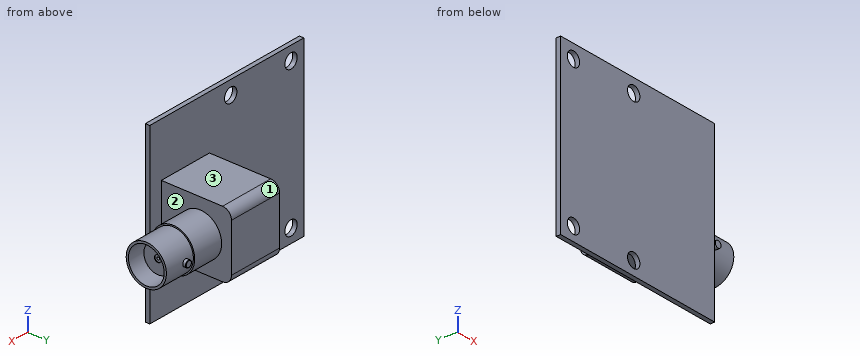
Autodesk Inventor part; units mm, degrees
ref_plane "YZ Plane" through (0, 0, 0) normal (1, 0, 0) x (0, 1, 0)
ref_plane "XZ Plane" through (0, 0, 0) normal (0, 1, 0) x (-1, 0, 0)
ref_plane "XY Plane" through (0, 0, 0) normal (0, 0, 1) x (1, 0, 0)
sketch "Sketch1" plane through (0, 0, 0) normal (0, 1, 0) x (-1, 0, 0)
  line L0 (0, 0) -> (40, 0)
  line L1 (40, 0) -> (40, -38.6)
  line L2 (40, -38.6) -> (0, -38.6)
  line L3 (0, -38.6) -> (0, 0)
  dimension "d0" = 40
  dimension "d1" = 38.6
extrude "Extrusion1" add sketch "Sketch1" along normal blind 1
sketch "Sketch6" plane through (0, 1, 0) normal (0, 1, 0) x (1, 0, 0)
  circle A0 centre (-36.676, 3.059) radius 1.6
  circle A1 centre (-21.026, 3.059) radius 1.6
  circle A2 centre (-21.026, 35.541) radius 1.6
  circle A3 centre (-36.676, 35.541) radius 1.6
  line L0 (0, 38.6) -> (-40, 38.6)
  line L1 (-40, 38.6) -> (-40, 0)
  point P0 (0, 0)
  dimension "d35" = 3.2
  dimension "d36" = 3.2
  dimension "d37" = 3.2
  dimension "d38" = 3.2
  dimension "d39" = 15.65
  dimension "d40" = 15.65
  dimension "d41" = 32.482
  dimension "d42" = 0
  dimension "d43" = 0
  dimension "d44" = 0
  dimension "d45" = 3.059
  dimension "d46" = 3.324
extrude "Extrusion5" cut sketch "Sketch6" against normal blind 5
sketch "Sketch7" plane through (0, 1, 0) normal (0, 1, 0) x (1, 0, 0)
  line L0 (-15.5, 26.65) -> (-3, 26.65)
  line L1 (-3, 26.65) -> (-3, 11.95)
  line L2 (-3, 11.95) -> (-15.5, 11.95)
  line L3 (-15.5, 11.95) -> (-15.5, 26.65)
  line L4 (0, 38.6) -> (-40, 38.6)
  line L5 (0, 0) -> (0, 38.6)
  dimension "d49" = 12.5
  dimension "d50" = 14.7
  dimension "d51" = 11.95
  dimension "d52" = 3
extrude "Extrusion6" add sketch "Sketch7" along normal blind 15.7
sketch "Sketch9" plane through (-3, 1, -11.95) normal (1, 0, 0) x (0, 0, -1)
  circle A0 centre (7.35, 8.7) radius 4.8
  line L0 (14.7, 0) -> (14.7, 15.7)
  line L1 (0, 15.7) -> (14.7, 15.7)
  point P0 (-11.95, -1)
  dimension "d55" = 9.6
  dimension "d56" = 7.35
  dimension "d57" = 7
extrude "Extrusion7" add sketch "Sketch9" along normal blind 7
fillet "Fillet1" radius 2 2 edges at (-9.25, 16.7, -11.95) (-9.25, 16.7, -26.65)
sketch "Sketch10" plane through (4, 9.7, -19.3) normal (1, 0, 0) x (0, 0, -1)
  circle A0 centre (0, 0) radius 4.5
  line L0 (7.35, -8.7) -> (7.35, 5)
  line L1 (-5.35, 7) -> (5.35, 7)
  point P0 (-19.3, -9.7)
  dimension "d61" = 9
  dimension "d62" = 7.35
  dimension "d63" = 7
extrude "Extrusion8" add sketch "Sketch10" along normal blind 7
sketch "Sketch11" plane through (11, 9.7, -19.3) normal (1, 0, 0) x (0, 0, -1)
  circle A0 centre (0, 0) radius 4
  point P0 (-19.3, -9.7)
  dimension "d66" = 8
extrude "Extrusion9" cut sketch "Sketch11" against normal blind 10
sketch "Sketch12" plane through (1, 9.7, -19.3) normal (1, 0, 0) x (0, 0, -1)
  circle A0 centre (0, 0) radius 3.1326
  point P0 (-19.3, -9.7)
extrude "Extrusion10" add sketch "Sketch12" along normal blind 7
sketch "Sketch13" plane through (8, 9.7, -19.3) normal (1, 0, 0) x (0, 0, -1)
  circle A0 centre (0, 0) radius 0.75
  point P0 (-19.3, -9.7)
  dimension "d75" = 1.5
extrude "Extrusion11" cut sketch "Sketch13" against normal blind 0.1
sketch "Sketch14" plane through (7.9, 9.7, -19.3) normal (1, 0, 0) x (0, 0, -1)
  circle A0 centre (0, 0) radius 0.2778
  point P0 (-19.3, -9.7)
extrude "Extrusion12" cut sketch "Sketch14" against normal blind 10
sketch "Sketch15" plane through (0, 16.7, 0) normal (0, 1, 0) x (1, 0, 0)
  circle A0 centre (6, 19.3) radius 0.75
  line L0 (-3, 26.65) -> (-15.5, 26.65)
  line L1 (-3, 13.95) -> (-3, 24.65)
  point P0 (0, 0)
  dimension "d76" = 1.5
  dimension "d77" = 7.35
  dimension "d78" = 9
extrude "Extrusion13" add sketch "Sketch15" against normal blind 20
sketch "Sketch16" plane through (6, 16.7, -19.3) normal (0, 1, 0) x (1, 0, 0)
  circle A0 centre (0, 0) radius 0.75
  point P0 (-6, -19.3)
extrude "Extrusion14" cut sketch "Sketch16" against normal blind 1.8
sketch "Sketch17" plane through (6, -3.3, -19.3) normal (0, -1, 0) x (1, 0, 0)
  circle A0 centre (0, 0) radius 0.75
  point P0 (-6, 19.3)
extrude "Extrusion15" cut sketch "Sketch17" against normal blind 7.7
fillet "Fillet2" radius 0.1 1 edges at (5.25, 14.9, -19.3)
properties part number "LED8"
Build history of the part. All positions in model axes, mm. Face numbers are marked on the shaded views. Round coordinates to 2 decimals unless told otherwise and drop trailing zeros. Loops run counter-clockwise (first coordinate to the right, second up) from the corner with the lowest first, then second, coordinate; pieces in that order, holes last. Notation, with made-up numbers: M 77.25,86.25 L 113.25,86.25 A10 cw 113.25,102.25 Z; hole C -2.5,31 d4. An arc over 180 degrees is marked long. Answer as CSV lines item,"result".
1. Flat gauge pins, fed straight in: P1, Ø4, axis at x = -9.5, y = 11, coming from the +Z side; P2, Ø3.5, axis at x = -36.676, z = -35.541, coming from the +Y side; P3, Ø1.4, axis at x = 6, z = -19.5, coming from the +Y side. Where does each tip first touch, or does it go through?
Resolved:
P1,"stops at z = -11.95"
P2,"stops at y = 1"
P3,"stops at y = 14.9"
2. Cut at A-A on z = -2.5. Write the cut outline in (x, y).
Resolved:
outline,"M -40,0 L -38.18,0 L -38.18,1 L -40,1 Z; M -35.18,0 L -22.53,0 L -22.53,1 L -35.18,1 Z; M -19.53,0 L 0,0 L 0,1 L -19.53,1 Z"
3. Cut at D-D on y = 11.75. Write the cut outline in (x, z).
Resolved:
outline,"M -15.5,-26.65 L -3,-26.65 L -3,-23.64 L 4,-23.64 L 4,-23.31 L 11,-23.31 L 11,-22.73 L 1,-22.73 L 1,-21.67 L 8,-21.67 L 8,-16.93 L 1,-16.93 L 1,-15.87 L 11,-15.87 L 11,-15.29 L 4,-15.29 L 4,-14.96 L -3,-14.96 L -3,-11.95 L -15.5,-11.95 Z"
4. Cut at B-B on x = 6. Write the cut outline in (y, z), then the cut area to 3 significant figures.
Resolved:
outline,"M 4.4,-20.05 L 5.26,-20.05 A4.5 ccw 14.14,-20.05 L 14.8,-20.05 A0.1 ccw 14.9,-19.95 L 14.9,-18.65 A0.1 ccw 14.8,-18.55 L 14.14,-18.55 A4.5 ccw 5.26,-18.55 L 4.4,-18.55 Z; hole M 5.77,-20.05 A4 ccw 13.63,-20.05 L 12.74,-20.05 A3.13 cw 6.66,-20.05 Z; hole M 5.77,-18.55 L 6.66,-18.55 A3.13 cw 12.74,-18.55 L 13.63,-18.55 A4 ccw Z"
area,"49.1 mm²"
5. Cut at C-C on z = -9. Write the cut outline in (x, y), then the cut area to 3 significant figures.
Resolved:
outline,"M -40,0 L 0,0 L 0,1 L -40,1 Z"
area,"40.0 mm²"
6. Wall check: probe 1 along Y at (x, z) = (7.25, -19.3); probe 2 along Y at (x, z) = (5.5, -18); probe 3 along Y at (x, z) = (-27.5, -22.5). Give the ranges that are in metal, low to high. Write a range as [from, to].
Resolved:
probe 1,"y = [5.2, 5.7], [6.57, 9.42], [9.98, 12.83], [13.7, 14.2]"
probe 2,"y = [5.39, 5.92], [6.85, 12.55], [13.48, 14.01]"
probe 3,"y = [0, 1]"
7. Two-plate mould, pull along Y, no slides. Class the marked faces 1, 2 and 3: released by +Y, released by -Y, zero draft, split by the parting line, or undercut.
Resolved:
face 1,"released by +Y"
face 2,"undercut"
face 3,"zero draft"
